Part model, mm, in its own coordinate system. A direction names the side the tool comes from. Coordinates: 2 decimals unless noted, no trailing zeros. Loops run counter-clockwise (first coordinate to the right, second up) from the corner with the lowest first, then second, coordinate; pieces in that order, holes last. Notation, with made-up numbers: (-40, -35) - (7, -35) arc R20 cw to (7, 1) - close; hole circle Ø6 at (51.5, 34). An arc over 180 degrees is marked (long way). Answer as CSV lines item,"result".
from build123d import *

# Parameters (mm, degrees)
SKETCH1_W           = 60
SKETCH1_H           = 100
SKETCH1_W_2         = 3.5
SKETCH1_H_2         = 30
SKETCH1_H_3         = 20
BOSS_EXTRUDE1_DEPTH = 5
SKETCH2_W           = 58
SKETCH2_H           = 3.5
BOSS_EXTRUDE2_DEPTH = 10
SKETCH3_W           = 52
SKETCH3_H           = 3
BOSS_EXTRUDE3_DEPTH = 2
SKETCH4_R           = 2
BOSS_EXTRUDE4_DEPTH = 20
CUT_EXTRUDE1_DEPTH  = 64.442887702
SKETCH6_W           = 3
SKETCH6_H           = 2
BOSS_EXTRUDE5_DEPTH = 3
SKETCH7_W           = 3
SKETCH7_H           = 2
BOSS_EXTRUDE6_DEPTH = 3
SKETCH8_W           = 5
SKETCH8_H           = 100
BOSS_EXTRUDE7_DEPTH = 10
BOSS_EXTRUDE8_DEPTH = 10
SKETCH11_W          = 70
SKETCH11_H          = 8.980295192
CUT_EXTRUDE2_DEPTH  = 69.738635424


with BuildPart() as part:
    # Sketch1 → Boss-Extrude1 (new body)
    with BuildSketch(Plane.XY):
        Rectangle(SKETCH1_W, SKETCH1_H)
        with Locations((24.25, -20)):
            Rectangle(SKETCH1_W_2, SKETCH1_H_2, mode=Mode.SUBTRACT)
        with Locations((-24.25, -20)):
            Rectangle(SKETCH1_W_2, SKETCH1_H_2, mode=Mode.SUBTRACT)
        with Locations((24.25, 30)):
            Rectangle(SKETCH1_W_2, SKETCH1_H_3, mode=Mode.SUBTRACT)
        with Locations((-24.25, 30)):
            Rectangle(SKETCH1_W_2, SKETCH1_H_3, mode=Mode.SUBTRACT)
    extrude(amount=BOSS_EXTRUDE1_DEPTH)

    # Sketch2 → Boss-Extrude2 (add)
    with BuildSketch(Plane.XY.offset(5)):
        with Locations((0, 4.173976932)):
            Rectangle(SKETCH2_W, SKETCH2_H)
    extrude(amount=BOSS_EXTRUDE2_DEPTH)

    # Sketch3 → Boss-Extrude3 (add)
    with BuildSketch(Plane(origin=(0, 5.923976932, 0), x_dir=(1, 0, 0), z_dir=(0, 1, 0))):
        with Locations((0, -10.12126967)):
            Rectangle(SKETCH3_W, SKETCH3_H)
    extrude(amount=BOSS_EXTRUDE3_DEPTH)

    # Sketch4 → Boss-Extrude4 (add)
    with BuildSketch(Plane(origin=(0, 0, 0), x_dir=(-1, 0, 0), z_dir=(0, 0, -1))):
        with Locations((15, 0)):
            Circle(SKETCH4_R)
        with Locations((-15, 0)):
            Circle(SKETCH4_R)
    extrude(amount=BOSS_EXTRUDE4_DEPTH)

    # Sketch5 → Cut-Extrude1 (cut, through all)
    with BuildSketch(Plane.XY.offset(5)):
        with BuildLine():
            Line((-20, 35.923976932), (20, 35.923976932))
            ThreePointArc((20, 35.923976932), (21, 34.923976932), (20, 33.923976932))
            Line((20, 33.923976932), (-20, 33.923976932))
            ThreePointArc((-20, 33.923976932), (-21, 34.923976932), (-20, 35.923976932))
        make_face()
    extrude(amount=-CUT_EXTRUDE1_DEPTH, mode=Mode.SUBTRACT)

    # Sketch6 → Boss-Extrude5 (add)
    with BuildSketch(Plane(origin=(26, 0, 0), x_dir=(0, 0, -1), z_dir=(1, 0, 0))):
        with Locations((-10.12126967, 6.923976932)):
            Rectangle(SKETCH6_W, SKETCH6_H)
    extrude(amount=BOSS_EXTRUDE5_DEPTH)

    # Sketch7 → Boss-Extrude6 (add)
    with BuildSketch(Plane.ZY.offset(26)):
        with Locations((10.12126967, 6.923976932)):
            Rectangle(SKETCH7_W, SKETCH7_H)
    extrude(amount=BOSS_EXTRUDE6_DEPTH)

    # Sketch8 → Boss-Extrude7 (add)
    with BuildSketch(Plane(origin=(30, 0, 0), x_dir=(0, 0, -1), z_dir=(1, 0, 0))):
        with Locations((-2.5, 0)):
            Rectangle(SKETCH8_W, SKETCH8_H)
    extrude(amount=BOSS_EXTRUDE7_DEPTH)

    # Sketch9 → Boss-Extrude8 (add)
    with BuildSketch(Plane(origin=(29, 0, 0), x_dir=(0, 0, -1), z_dir=(1, 0, 0))):
        Polygon((-5, 2.423976932), (-5, 5.923976932), (-8.62126967, 5.923976932), (-8.62126967, 7.923976932), (-11.62126967, 7.923976932), (-11.62126967, 5.923976932), (-15, 5.923976932), (-15, 2.423976932), align=None)
    extrude(amount=BOSS_EXTRUDE8_DEPTH)

    # Sketch11 → Cut-Extrude2 (cut, through all)
    with BuildSketch(Plane.XY.offset(5)):
        with Locations((5, 45.509852404)):
            Rectangle(SKETCH11_W, SKETCH11_H)
    extrude(amount=-CUT_EXTRUDE2_DEPTH, mode=Mode.SUBTRACT)


solid = part.part
Q1. Wall check: L1, parallel to X at y = -6, z = 3; L2, parallel to Z at x = 28.5, y = -26; L3, parallel to X at y = 5, z = 12. Give the ranges that are in metal, low to high.
Results:
L1,"x = -30 to -26, -22.5 to 22.5, 26 to 40"
L2,"z = 0 to 5"
L3,"x = -29 to 39"
Q2. Saw through at A-A (y = -29.5). Give the cut face in (x, z), then the cut area to 3 significant figures.
Results:
outline,"(-30, 0) - (-26, 0) - (-26, 5) - (-30, 5) - close; (-22.5, 0) - (22.5, 0) - (22.5, 5) - (-22.5, 5) - close; (26, 0) - (40, 0) - (40, 5) - (26, 5) - close"
area,"315 mm^2"
Q3. Saw through at D-D (y = 0). Give the cut face in (x, z), then the cut area to 3 significant figures.
Results:
outline,"(-30, 0) - (-17, 0) - (-17, -20) - (-13, -20) - (-13, 0) - (13, 0) - (13, -20) - (17, -20) - (17, 0) - (40, 0) - (40, 5) - (-30, 5) - close"
area,"510 mm^2"
Q4. Flat gauge pins, fed straight in: pin 1 (6 mm diameter, centred on y = 5.5, z = 9.5, fed in from +X); pin 2 (2 mm diameter, centred on x = -16.5, y = -28, fed in from +Z); pin 3 (1 mm diameter, centred on x = -2.5, y = 7, fed in from +Z). Where does each tip first touch, or does it go through?
Results:
pin 1,"stops at x = 39"
pin 2,"stops at z = 5"
pin 3,"stops at z = 11.62"
Q5. Saw through at C-C (x = -4). Give the cut face in (y, z).
Results:
outline,"(-50, 0) - (33.92, 0) - (33.92, 5) - (5.92, 5) - (5.92, 8.62) - (7.92, 8.62) - (7.92, 11.62) - (5.92, 11.62) - (5.92, 15) - (2.42, 15) - (2.42, 5) - (-50, 5) - close; (35.92, 0) - (41.02, 0) - (41.02, 5) - (35.92, 5) - close"
Q6. Two-plate mould, pull along X, no slides. Class faces 1 (the face through (39, 5, 10)), 2 (the face through (26, 30, 2)), 3 (the face through (5, 4, 15)): released by +X, released by -X, zero draft, split by the parting line, or undercut.
Results:
face 1,"released by +X"
face 2,"undercut"
face 3,"zero draft"
Q7. Saw through at B-B (x = 24.5). Give the cut face in (y, z), then the cut area to 3 significant figures.
Results:
outline,"(-50, 0) - (-35, 0) - (-35, 5) - (-50, 5) - close; (-5, 0) - (20, 0) - (20, 5) - (5.92, 5) - (5.92, 8.62) - (7.92, 8.62) - (7.92, 11.62) - (5.92, 11.62) - (5.92, 15) - (2.42, 15) - (2.42, 5) - (-5, 5) - close; (40, 0) - (41.02, 0) - (41.02, 5) - (40, 5) - close"
area,"246 mm^2"
Q8. Which spindle directions (+Z, -Z, +X, -X, +Y, -Y) get a long thin tool onto all of the face, cutting with end or side? Do faces 4 (the face through (5, 7, 8.621)), 5 (the face through (16.6, -1.2, -9.9)), 6 (the face through (22.5, -20, 2)), 7 (the face through (5, 2.424, 10)). Say none if no direction does.
Results:
face 4,"+X, -X, +Y"
face 5,"-Z"
face 6,"+Z, -Z"
face 7,"+Z, +X, -X, -Y"
